```python
from build123d import *

# Parameters (mm, degrees)
PAD008_DEPTH    = 10
SKETCH029_R     = 3.175
POCKET018_DEPTH = 187.8463782794
POCKET019_DEPTH = 187.8463789695
POCKET020_DEPTH = 19
PAD009_DEPTH    = 20
CHAMFER007_SIZE = 3
CHAMFER008_SIZE = 1
FILLET002_R     = 3


with BuildPart() as part:
    # Sketch028 → Pad008 (new body, symmetric)
    with BuildSketch(Plane.XY):
        with BuildLine():
            ThreePointArc((0, 19.3), (-19.3, 0), (0, -19.3))
            Line((0, -19.3), (0, -37.3))
            ThreePointArc((0, 37.3), (-25.3, 0), (0, -37.3))
            Line((0, 37.3), (0, 19.3))
        make_face()
    extrude(amount=PAD008_DEPTH, both=True)

    # Sketch029 (on Face3 of Pad008) → Pocket018 (cut, through all)
    with BuildSketch(Plane.YZ):
        with Locations((-31.3, 0)):
            Circle(SKETCH029_R)
    pocket018 = extrude(amount=-POCKET018_DEPTH, mode=Mode.SUBTRACT)

    # Mirrored018: Pocket018 across Sketch029 V_Axis
    add(pocket018.mirror(Plane(origin=(0, 0, 0), x_dir=(1, 0, 0), z_dir=(0, 1, 0))), mode=Mode.SUBTRACT)

    # Sketch030 (on Face7 of Mirrored018) → Pocket019 (cut, through all)
    with BuildSketch(Plane.YZ):
        Polygon((-32.3, 3.0134075396), (-30.3, 3.0134075396), (-30.55, 3.2634075396), (-32.05, 3.2634075396), align=None)
    pocket019 = extrude(amount=-POCKET019_DEPTH, mode=Mode.SUBTRACT)

    # Mirrored019: Pocket019 across Sketch030 V_Axis
    add(pocket019.mirror(Plane(origin=(0, 0, 0), x_dir=(1, 0, 0), z_dir=(0, 1, 0))), mode=Mode.SUBTRACT)

    # Sketch031 (on DatumPlane) → Pocket020 (cut)
    with BuildSketch(Plane(origin=(-25, 0, 0), x_dir=(0, -1, 0), z_dir=(-1, 0, 0))):
        Polygon((25.7, -3.2331615075), (25.7, 10), (37.3, 10), (37.3, -6.4663230149), (31.3, -6.4663230149), align=None)
    pocket020 = extrude(amount=-POCKET020_DEPTH, mode=Mode.SUBTRACT)

    # Mirrored020: Pocket020 across Sketch031 V_Axis
    add(pocket020.mirror(Plane(origin=(-25, 0, 0), x_dir=(-1, 0, 0), z_dir=(0, -1, 0))), mode=Mode.SUBTRACT)

    # Sketch032 (on Face4 of Mirrored020) → Pad009 (join)
    with BuildSketch(Plane.XY.offset(10)):
        Polygon((0, -37.3), (-6, -37.3), (-6, -34.3094710302), align=None)
    pad009 = extrude(amount=-PAD009_DEPTH)

    # Mirrored021: Pad009 across Sketch032 H_Axis
    add(pad009.mirror(Plane(origin=(0, 0, 10), x_dir=(0, 0, 1), z_dir=(0, 1, 0))))

    # Chamfer007
    chamfer007_edges = [part.edges().sort_by_distance(p)[0] for p in [
        (-3, -37.3, 10),
        (-25.3, 0, 10),
        (-3, 37.3, 10),
    ]]
    chamfer(chamfer007_edges, length=CHAMFER007_SIZE)

    # Chamfer008
    chamfer008_edges = [part.edges().sort_by_distance(p)[0] for p in [
        (-6, -37.3, -1.5),
        (-6, -35.8, 8.5),
        (-6, -30, 10),
        (-8.987185, -25.7, 10),
        (-13.996133, -25.7, 8.514904),
        (-15.995669, -25.7, 1.883419),
        (-15.995669, 25.7, 1.883419),
        (-13.996133, 25.7, 8.514904),
        (-8.987185, 25.7, 10),
        (-6, 30, 10),
        (-6, 35.8, 8.5),
        (-6, 37.3, -1.5),
    ]]
    chamfer(chamfer008_edges, length=CHAMFER008_SIZE)

    # Fillet002
    fillet002_edges = [part.edges().sort_by_distance(p)[0] for p in [
        (-6, 34.309471, -8.233162),
        (-6, -34.309471, -8.233162),
    ]]
    fillet(fillet002_edges, radius=FILLET002_R)


solid = part.part
```
Source: CAD feature listing. Evaluate the final solid. Frame: model axes, mm. A direction names the side the tool comes from. Coordinates: 2 decimals unless noted, no trailing zeros. Write each loop counter-clockwise with the first axis right and the second up, starting at its lowest first coordinate (ties: lowest second). Pieces come first, ordered by that corner, then holes. Notation, with made-up numbers: (-31.5, 38.25) - (-2.5, 38.25) arc R19 cw to (-2.5, 63.25) - close; hole circle Ø8 at (-27, -19.5). An arc over 180 degrees is marked (long way). Answer as a JSON object with one key per item and string values.
Q1. Set-up query: faces 1 (the flat face through (-15.8, -25.317, 1.727)), 2 (the flat face through (-6, 31, 4)), 3 (the flat face through (0, 26, 0)). Return all of +Z, -Z, +X, -X, +Y, -Y with unobstructed straight access to the full face (end or side cutting, diameter ignored); none if empty.
Ans:
{"face 1": "+Z, -X, -Y", "face 2": "+Z, -X, +Y", "face 3": "+Z, -Z, +X, +Y, -Y"}
Q2. Section query B-B, the plane y = 0. Output: boundary loops of the cut face in (x, z), plus the area to 4 significant figures.
Ans:
{"outline": "(-25.3, -10) - (-19.3, -10) - (-19.3, 10) - (-22.3, 10) - (-25.3, 7) - close", "area": "115.5 mm2"}
Q3. Section query A-A, the plane z = 0. Output: boundary loops of the cut face in (x, y) (3 decimals), plus the area to 3 significant figures.
Ans:
{"outline": "(-16.626, -24.924) - (-14.996, -25.7) - (-6, -25.7) - (-6, -28.125) - (0, -28.125) - (0, -19.3) arc R19.3 cw to (0, 19.3) - (0, 28.125) - (-6, 28.125) - (-6, 25.7) - (-14.996, 25.7) - (-16.626, 24.924) arc R40.146 ccw to start; (-6, -36.3) - (-5, -37.3) - (0, -37.3) - (0, -34.475) - (-5.668, -34.475) - (-6, -34.309) - close; (-6, 34.309) - (-5.668, 34.475) - (0, 34.475) - (0, 37.3) - (-5, 37.3) - (-6, 36.3) - close", "area": "625 mm2"}
Q4. Draft query along Z for faces 4 (the cylindrical face through (-2.958, -31.425, -3.173)), 5 (the conical face through (-22.444, 0.381, 9.854)), 6 (the flat face through (-15.8, 25.317, 1.727)). Return one class per face: released by +Z, released by -Z, zero draft, split by the parting line, or undercut.
Ans:
{"face 4": "undercut", "face 5": "released by +Z", "face 6": "zero draft"}
Q5. Section query D-D, the plane z = -8.25. Output: boundary loops of the cut face in (x, y).
Ans:
{"outline": "(-7.34, -33.46) arc R3 cw to (-6, -35.96) - (-6, -36.3) - (-5, -37.3) - (0, -37.3) - (0, -19.3) arc R19.3 cw to (0, 19.3) - (0, 37.3) - (-5, 37.3) - (-6, 36.3) - (-6, 35.96) arc R3 cw to (-7.34, 33.46) arc R40.15 ccw to start"}
Q6. Material intervals for line 1 (Z direction, x = -4.5, y = 31.3) (3 decimals); line 2 (Y direction, x = -4.5, z = 0) (3 decimals); line 3 (Y direction, x = -1.5, z = 0) (3 decimals), sorted ascending. Write a range as [from, to].
Ans:
{"line 1": "z = [-10, -3.175], [3.263, 10]", "line 2": "y = [-37.3, -34.475], [-28.125, -18.768], [18.768, 28.125], [34.475, 37.3]", "line 3": "y = [-37.3, -34.475], [-28.125, -19.242], [19.242, 28.125], [34.475, 37.3]"}
Q7. Section query C-C, the plane x = -9.5. Output: boundary loops of the cut face in (y, z), plus the area to 3 significant figures.
Ans:
{"outline": "(-31.92, -10) - (-16.8, -10) - (-16.8, 10) - (-24.7, 10) - (-25.7, 9) - (-25.7, -3.23) - (-31.3, -6.47) - (-31.92, -6.47) - close; (16.8, -10) - (31.92, -10) - (31.92, -6.47) - (31.3, -6.47) - (25.7, -3.23) - (25.7, 9) - (24.7, 10) - (16.8, 10) - close", "area": "417 mm2"}
Q8. First-contact query: pin 1 Ø11.5 at (y, z) = (29.5, -4.5) entering from -X; pin 2 Ø3.5 at (x, y) = (-8.5, -33.5) entering from +Z; pin 3 Ø8 at (y, z) = (8, -1.5) entering from -X. Flat tips, straight axial feed; report the tip coordinate or a pass-through.
Ans:
{"pin 1": "stops at x = -17.52", "pin 2": "stops at z = -6.47", "pin 3": "stops at x = -25.1"}
